from build123d import *

# Parameters (mm, degrees)
F0_W     = 160
F0_H     = 40
F0_R     = 3
F1_DEPTH = 7
F2_SIZE  = 3


with BuildPart() as f1:
    # F0 (on Top) → F1 (new body)
    with BuildSketch(Plane.XY):
        with Locations((80, 20)):
            Rectangle(F0_W, F0_H)
        with Locations((10, 10)):
            Circle(F0_R, mode=Mode.SUBTRACT)
        with Locations((111.5, 9)):
            Circle(F0_R, mode=Mode.SUBTRACT)
        with Locations((133.5, 9)):
            Circle(F0_R, mode=Mode.SUBTRACT)
        with Locations((150, 10)):
            Circle(F0_R, mode=Mode.SUBTRACT)
        with Locations((10, 30)):
            Circle(F0_R, mode=Mode.SUBTRACT)
        with Locations((111.5, 31)):
            Circle(F0_R, mode=Mode.SUBTRACT)
        with Locations((133.5, 31)):
            Circle(F0_R, mode=Mode.SUBTRACT)
        with Locations((150, 30)):
            Circle(F0_R, mode=Mode.SUBTRACT)
    extrude(amount=F1_DEPTH)

    # F2
    f2_edges = [f1.edges().sort_by_distance(p)[0] for p in [
        (108.5, 31, 7),
        (130.5, 31, 7),
        (130.5, 9, 7),
        (108.5, 9, 7),
        (147, 10, 0),
        (147, 30, 0),
        (7, 10, 0),
        (7, 30, 0),
    ]]
    chamfer(f2_edges, length=F2_SIZE)


solid = f1.part
The listing builds one solid part. Answer for the finished solid, in the listing's coordinates (mm). Round coordinates to 2 decimals unless told otherwise and drop trailing zeros. Loops run counter-clockwise (first coordinate to the right, second up) from the corner with the lowest first, then second, coordinate; pieces in that order, holes last. Notation, with made-up numbers: M 2,44.5 L 37,44.5 A22 cw 37,80.5 Z; hole C 25,1.25 d8. An arc over 180 degrees is marked long. Return JSON: item names as keys, results as strings.
Q1. Each of these flat-tipped pins is pushed along its axis until it touches: pin 1 Ø8 at (x, y) = (10, 10) entering from -Z; pin 2 Ø9.5 at (x, y) = (133.5, 9) entering from +Z. Where does it stop, or does it pass through?
Results list:
{"pin 1": "stops at z = 2", "pin 2": "stops at z = 5.75"}
Q2. Find section B-B, the plane z = 1.25. State how many separate pieces and enclosed holes the cut face has, plus the area to 3 significant figures.
Results list:
{"separate pieces": "1", "enclosed holes": "8", "area": "6,000 mm2"}
Q3. The mould has two halves that part along X. Classify faces 1 (the face through (160, 20, 3)), 2 (the face through (79, 20, 0)), 3 (the face through (114.36, 9.9, 1.97)), 4 (the face through (0, 20, 3)): released by +X, released by -X, zero draft, split by the parting line, or undercut.
Results list:
{"face 1": "released by +X", "face 2": "zero draft", "face 3": "undercut", "face 4": "released by -X"}
Q4. Find section A-A, the plane x = 111.5. Determine the outline of the cut face in (y, z).
Results list:
{"outline": "M 0,0 L 6,0 L 6,4 L 3,7 L 0,7 Z; M 12,0 L 28,0 L 28,4 L 25,7 L 15,7 L 12,4 Z; M 34,0 L 40,0 L 40,7 L 37,7 L 34,4 Z"}
Q5. Find the intervals of material crossed by line 1 along Y through (x, z) = (10, 5.1); line 2 along X through (y, z) = (34, 5.25); line 3 along Y through (x, z) = (132, 2.75), in increasing order. Write a range as from..to.
Results list:
{"line 1": "y = 0..7, 13..27, 33..40", "line 2": "x = 0..108.49, 114.51..130.49, 136.51..160", "line 3": "y = 0..6.4, 11.6..28.4, 33.6..40"}
